```python
from build123d import *

# Parameters (mm, degrees)
BOSS_EXTRUDE1_DEPTH            = 20
CBORE_FOR_M5_SHCS1_D           = 5.5
CBORE_FOR_M5_SHCS1_CBORE_D     = 10
CBORE_FOR_M5_SHCS1_CBORE_DEPTH = 65
SKETCH5_W                      = 8
SKETCH5_H                      = 6.1
BOSS_EXTRUDE2_DEPTH            = 4
SKETCH6_R                      = 1.4
CUT_EXTRUDE1_DEPTH             = 21
FILLET1_R                      = 5
CHAMFER2_SIZE                  = 1


with BuildPart() as part:
    # Sketch1 → Boss-Extrude1 (new body)
    with BuildSketch(Plane(origin=(0, 0, 0), x_dir=(1, 0, 0), z_dir=(0, 1, 0))):
        Polygon((0, 0), (0, 71.12), (25, 71.12), (25, 61.12), (15, 61.12), (15, 10), (25, 10), (25, 0), align=None)
    extrude(amount=BOSS_EXTRUDE1_DEPTH)

    # CBORE for M5 SHCS1 (through all)
    with Locations(Plane(origin=(0, 0, -71.12), x_dir=(-1, 0, 0), z_dir=(0, 0, -1))):
        with Locations((-7.5, 10)):
            CounterBoreHole(CBORE_FOR_M5_SHCS1_D / 2, CBORE_FOR_M5_SHCS1_CBORE_D / 2, CBORE_FOR_M5_SHCS1_CBORE_DEPTH)

    # Sketch5 → Boss-Extrude2 (add)
    with BuildSketch(Plane.XY):
        with Locations((21, 10)):
            Rectangle(SKETCH5_W, SKETCH5_H)
    extrude(amount=BOSS_EXTRUDE2_DEPTH)

    # Sketch6 → Cut-Extrude1 (cut, through all)
    with BuildSketch(Plane.XZ):
        with Locations((18.81, -3.81)):
            Circle(SKETCH6_R)
        with Locations((18.81, -66.04)):
            Circle(SKETCH6_R)
    extrude(amount=-CUT_EXTRUDE1_DEPTH, mode=Mode.SUBTRACT)

    # Fillet1
    fillet1_edges = [part.edges().sort_by_distance(p)[0] for p in [
        (25, 10, -61.12),
        (25, 10, -10),
    ]]
    fillet(fillet1_edges, radius=FILLET1_R)

    # Chamfer2
    chamfer2_edges = [part.edges().sort_by_distance(p)[0] for p in [
        (15, 0, -35.56),
        (25, 0, -2.5),
        (12.5, 0, 0),
        (15, 20, -35.56),
        (17.5, 20, -61.12),
        (12.5, 20, -71.12),
        (0, 20, -35.56),
        (17.41, 20, -3.81),
        (17.41, 0, -3.81),
        (17.41, 20, -66.04),
        (17.41, 0, -66.04),
        (12.5, 20, 0),
        (17.5, 0, -10),
        (17.5, 20, -10),
        (25, 0, -68.62),
        (23.535533906, 0, -62.584466094),
        (23.535533906, 0, -8.535533906),
        (25, 20, -68.62),
        (23.535533906, 20, -62.584466094),
        (23.535533906, 20, -8.535533906),
        (0, 0, -35.56),
        (25, 20, -2.5),
        (12.5, 0, -71.12),
        (17.5, 0, -61.12),
    ]]
    chamfer(chamfer2_edges, length=CHAMFER2_SIZE)


solid = part.part
```
For this review, take the finished solid that the model builds, in its own axes (mm). A direction names the side the tool comes from. Round coordinates to 2 decimals unless told otherwise and drop trailing zeros. Write each loop counter-clockwise with the first axis right and the second up, starting at its lowest first coordinate (ties: lowest second). Pieces come first, ordered by that corner, then holes. Notation, with made-up numbers: (54.25, 79.25) -> (106.25, 79.25) arc R24 ccw to (106.25, 89.25) -> close; hole circle Ø8 at (-36.75, -32.75). An arc over 180 degrees is marked (long way). One line per question, with ' | ' between items. Start each with the question number.
(1) Add section C-C, the plane x = 7.5. Write out the cut boundary in (y, z), plus the area to 3 significant figures.
(2) Insertion check: P1, Ø5.5, axis at y = 7.5, z = -31, coming from the +X side; P2, Ø4.5, axis at x = 22, z = 3, coming from the +Y side; P3, Ø3, axis at x = 7.5, y = 3, coming from the +Z side. Each pin has a flat end and moves straight along its axis. Give the tip position at first contact, or say it passes through.
(3) Add section D-D, the plane y = 14. Write out the cut boundary in (x, z).
(4) Mouldability with a two-part tool opening along Y and no side actions: class faces 5 (the face through (18.63, 9.87, -64.65)), 6 (the face through (22.996, 0.285, -8.063)), 7 (the face through (5, 8, -6.12)), 8 (the face through (10.12, 10.83, -3.02)) as released by +Y, released by -Y, zero draft, split by the parting line, or undercut.
(5) For line 1 along X through (y, z) = (13, -67); line 2 along Z through (x, y) = (18, 11.5); line 3 along Y through (x, z) = (7.5, -2), list the stretches that pass through material, from the lowest coordinate up. Write a range as from..to.
(6) Add section B-B, the plane z = -3.81. Write out the cut boundary in (x, y), plus the area to 3 significant figures.
(7) Add section A-A, the plane y = 10. Write out the cut boundary in (x, z), plus the area to 3 significant figures.
(8) Tool access review of faces 1 (the face through (22.99, 19.73, -8.05)), 2 (the face through (23.57, 10.13, -62.62)), 3 (the face through (17, 10, 2)), 4 (the face through (23.063, 0.285, -63.124)): name each direction out of +Z, -Z, +X, -X, +Y, -Y from which nothing blocks a thin tool from reaching the whole face with its end or side.
Answer list:
1) outline: (0, -70.12) -> (1, -71.12) -> (5, -71.12) -> (5, -6.12) -> (7.25, -6.12) -> (7.25, 0) -> (1, 0) -> (0, -1) -> close; (12.75, -6.12) -> (15, -6.12) -> (15, -71.12) -> (19, -71.12) -> (20, -70.12) -> (20, -1) -> (19, 0) -> (12.75, 0) -> close | area: 737 mm²
2) P1: x = 15 | P2: y = 13.05 | P3: z = 0
3) outline: (0, -71.12) -> (4.5, -71.12) -> (4.5, -6.12) -> (10.5, -6.12) -> (10.5, -71.12) -> (25, -71.12) -> (25, -66.12) arc R5 ccw to (20, -61.12) -> (15, -61.12) -> (15, -10) -> (20, -10) arc R5 ccw to (25, -5) -> (25, 0) -> (0, 0) -> close; hole circle Ø2.8 at (18.81, -66.04); hole circle Ø2.8 at (18.81, -3.81)
4) face 5: zero draft | face 6: released by -Y | face 7: undercut | face 8: undercut
5) line 1: 0..3.5, 11.5..17.79, 19.83..25 | line 2: -71.12..-67.18, -64.9..-61.12, -10..-4.95, -2.67..4 | line 3: 0..7.25, 12.75..20
6) outline: (0, 1) -> (1, 0) -> (16.41, 0) -> (17.41, 1) -> (17.41, 19) -> (16.41, 20) -> (1, 20) -> (0, 19) -> close; (20.21, 1) -> (21.21, 0) -> (24, 0) -> (25, 1) -> (25, 19) -> (24, 20) -> (21.21, 20) -> (20.21, 19) -> close; hole circle Ø5.5 at (7.5, 10) | area: 416 mm²
7) outline: (0, -71.12) -> (2.5, -71.12) -> (2.5, -6.12) -> (4.75, -6.12) -> (4.75, 0) -> (0, 0) -> close; (10.25, -6.12) -> (12.5, -6.12) -> (12.5, -71.12) -> (25, -71.12) -> (25, -66.12) arc R5 ccw to (20, -61.12) -> (15, -61.12) -> (15, -10) -> (20, -10) arc R5 ccw to (25, -5) -> (25, 4) -> (17, 4) -> (17, 0) -> (10.25, 0) -> close; hole circle Ø2.8 at (18.81, -66.04); hole circle Ø2.8 at (18.81, -3.81) | area: 592 mm²
8) face 1: +X, +Y | face 2: +X, +Y, -Y | face 3: +Z, -X, +Y, -Y | face 4: +X, -Y
